from build123d import *

# Parameters (mm, degrees)
BOSS_EXTRUDE1_DEPTH = 3.175
CUT_EXTRUDE1_DEPTH  = 267.323293548


with BuildPart() as part:
    # Sketch1 → Boss-Extrude1 (new, symmetric)
    with BuildSketch(Plane.XY):
        Polygon((-130.838522478, 95.25), (-29.238522478, 95.25), (-29.238522478, 231.881554295), (-130.838522478, 173.222766945), align=None)
    extrude(amount=BOSS_EXTRUDE1_DEPTH, both=True)

    # Sketch2 → Cut-Extrude1 (cut, through all)
    with BuildSketch(Plane.XY.offset(3.175)):
        Polygon((-54.638522478, 120.65), (-54.638522478, 187.887463782), (-105.438522478, 158.558070107), (-105.438522478, 120.65), align=None)
    extrude(amount=-CUT_EXTRUDE1_DEPTH, mode=Mode.SUBTRACT)


solid = part.part
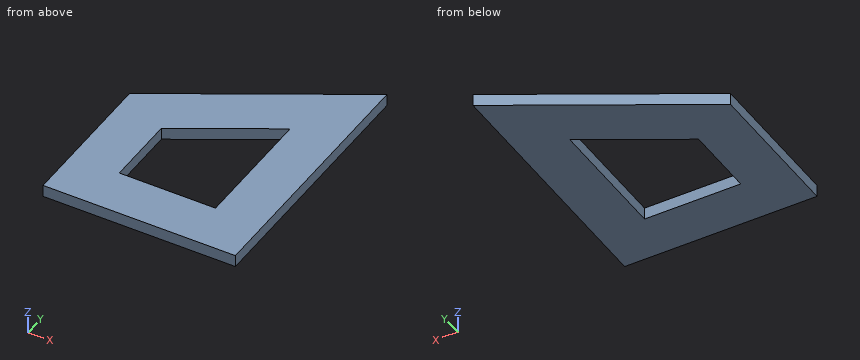
CAD build for the part. Positions are in the model's coordinates, mm. Round coordinates to 2 decimals unless told otherwise and drop trailing zeros. Order: outer loops, then holes, each group sorted by start corner. A loop starts at its lowest first (then second) coordinate and runs counter-clockwise, first axis right, second up. Notation, with made-up numbers: (76, -25.5) -> (93, -25.5) arc R16 cw to (93, -21.5) -> close; hole circle Ø7 at (35.25, 41). An arc over 180 degrees is marked (long way). Write each question's results on one line, items separated by ' | '.
1. Cut at B-B (x = -80.5). Give the cut face in (y, z) (3 decimals).
Findings below:
outline: (95.25, -3.175) -> (120.65, -3.175) -> (120.65, 3.175) -> (95.25, 3.175) -> close; (172.956, -3.175) -> (202.286, -3.175) -> (202.286, 3.175) -> (172.956, 3.175) -> close
2. Cut at A-A (y = 132). Give the cut face in (x, z) (3 decimals).
Findings below:
outline: (-130.839, -3.175) -> (-105.439, -3.175) -> (-105.439, 3.175) -> (-130.839, 3.175) -> close; (-54.639, -3.175) -> (-29.239, -3.175) -> (-29.239, 3.175) -> (-54.639, 3.175) -> close
3. Flat gauge pins, fed straight in: P1, Ø3, axis at x = -93.5, z = -0.5, coming from the +Y side; P2, Ø3, axis at x = -56.5, z = 0, coming from the +Y side. Where does each tip first touch, or does it go through?
Findings below:
P1: stops at y = 195.65 | P2: stops at y = 217.01
4. Wall check: line 1 along X through (y, z) = (140.5, 2); line 2 along Y through (x, z) = (-96, 0.25); line 3 along Y through (x, z) = (-80.5, -2.25). Give the ranges that are in metal, low to high. Write a range as [from, to].
Findings below:
line 1: x = [-130.84, -105.44], [-54.64, -29.24] | line 2: y = [95.25, 120.65], [164.01, 193.34] | line 3: y = [95.25, 120.65], [172.96, 202.29]
5. Cut at D-D (x = -117). Give the cut face in (y, z) (3 decimals), plus the area to 3 significant figures.
Findings below:
outline: (95.25, -3.175) -> (181.212, -3.175) -> (181.212, 3.175) -> (95.25, 3.175) -> close | area: 546 mm²
6. Cut at C-C (z = 1.25). Give the cut face in (x, y).
Findings below:
outline: (-130.84, 95.25) -> (-29.24, 95.25) -> (-29.24, 231.88) -> (-130.84, 173.22) -> close; hole (-105.44, 120.65) -> (-54.64, 120.65) -> (-54.64, 187.89) -> (-105.44, 158.56) -> close
